Here's how the part is built. I have some questions about the finished solid (model axes, mm). Face numbers are marked on the shaded views. A direction names the side the tool comes from. Round coordinates to 2 decimals unless told otherwise and drop trailing zeros. Loops run counter-clockwise (first coordinate to the right, second up) from the corner with the lowest first, then second, coordinate; pieces in that order, holes last. Notation, with made-up numbers: (-0.75, 24.25) - (23.25, 24.25) arc R14 ccw to (23.25, 38.25) - close; hole circle Ø10 at (34, 70.5). An arc over 180 degrees is marked (long way). Answer as a JSON object with one key per item and string values. Group by question number.
1) Will these pins go through, and if not, where does the flat tip stop? P1, Ø1.8, axis at x = 6, z = 7, coming from the +Y side; P2, Ø6, axis at x = 10.5, y = 6, coming from the +Z side; P3, Ø1, axis at x = 2.5, z = 5.5, coming from the +Y side.
2) I want a section at C-C, the plane x = 5.95. Please give me the cut outline in (y, z).
3) If I drill on line 1 along Z through (x, y) = (7.5, 4.5); line 2 along Y through (x, z) = (7.25, 1.5); line 3 along Y through (x, z) = (5, 7), over which ranges is the centre line in solid material (lowest first)? Write a range as [from, to].
4) I want a section at B-B, the plane y = 3. Please give me the cut outline in (x, z), then the cut area to 3 significant figures.
5) I want a section at A-A, the plane x = 9.5. Please give me the cut outline in (y, z).
6) I want a section at D-D, the plane y = 5. Please give me the cut outline in (x, z), then the cut area to 3 significant figures.
7) Which directions (+Z, -Z, +X, -X, +Y, -Y) give clear straight access to the entire face, cutting with the end or side of a thin tool? Please do the marked faces 1 and 2.
from build123d import *

# Parameters (mm, degrees)
CROQUIS1_W              = 11.9
CROQUIS1_H              = 9.3
SALIENTE_EXTRUIR1_DEPTH = 10
SALIENTE_EXTRUIR2_DEPTH = 10
SALIENTE_EXTRUIR3_DEPTH = 16.3
CROQUIS6_W              = 10.1
CROQUIS6_H              = 0.1
CORTAR_EXTRUIR1_DEPTH   = 0.1
CROQUIS7_W              = 0.1
CROQUIS7_H              = 8.2
CORTAR_EXTRUIR2_DEPTH   = 0.1
CROQUIS8_W              = 0.1
CROQUIS8_H              = 8.2
CORTAR_EXTRUIR3_DEPTH   = 0.1
CROQUIS9_W              = 10.1
CROQUIS9_H              = 0.1
CORTAR_EXTRUIR4_DEPTH   = 0.1


with BuildPart() as part:
    # Croquis1 → Saliente-Extruir1 (new body)
    with BuildSketch(Plane(origin=(0, 0, 0), x_dir=(1, 0, 0), z_dir=(0, 1, 0))):
        with Locations((5.95, 4.65)):
            Rectangle(CROQUIS1_W, CROQUIS1_H)
    extrude(amount=SALIENTE_EXTRUIR1_DEPTH)

    # Croquis2 → Saliente-Extruir2 (add)
    with BuildSketch(Plane.XY):
        with BuildLine():
            Line((4.831966011, 6), (7.068033989, 6))
            ThreePointArc((7.068033989, 6), (5.95, 3.5), (4.831966011, 6))
        make_face()
    extrude(amount=SALIENTE_EXTRUIR2_DEPTH)

    # Croquis3 → Saliente-Extruir3 (add)
    with BuildSketch(Plane(origin=(0, 0, -9.3), x_dir=(-1, 0, 0), z_dir=(0, 0, -1))):
        with BuildLine():
            Line((-11, 10), (-0.9, 10))
            ThreePointArc((-0.9, 10), (-0.263603897, 9.736396103), (0, 9.1))
            Line((0, 9.1), (0, 0.9))
            ThreePointArc((0, 0.9), (-0.263603897, 0.263603897), (-0.9, 0))
            Line((-0.9, 0), (-11, 0))
            ThreePointArc((-11, 0), (-11.636396103, 0.263603897), (-11.9, 0.9))
            Line((-11.9, 0.9), (-11.9, 9.1))
            ThreePointArc((-11.9, 9.1), (-11.636396103, 9.736396103), (-11, 10))
        make_face()
    extrude(amount=SALIENTE_EXTRUIR3_DEPTH)

    # Croquis6 → Cortar-Extruir1 (cut)
    with BuildSketch(Plane(origin=(0, 10, 0), x_dir=(1, 0, 0), z_dir=(0, 1, 0))):
        with Locations((5.95, 9.35)):
            Rectangle(CROQUIS6_W, CROQUIS6_H)
    extrude(amount=-CORTAR_EXTRUIR1_DEPTH, mode=Mode.SUBTRACT)

    # Croquis7 → Cortar-Extruir2 (cut)
    with BuildSketch(Plane(origin=(11.9, 0, 0), x_dir=(0, 0, -1), z_dir=(1, 0, 0))):
        with Locations((9.35, 5)):
            Rectangle(CROQUIS7_W, CROQUIS7_H)
    extrude(amount=-CORTAR_EXTRUIR2_DEPTH, mode=Mode.SUBTRACT)

    # Croquis8 → Cortar-Extruir3 (cut)
    with BuildSketch(Plane.ZY):
        with Locations((-9.35, 5)):
            Rectangle(CROQUIS8_W, CROQUIS8_H)
    extrude(amount=-CORTAR_EXTRUIR3_DEPTH, mode=Mode.SUBTRACT)

    # Croquis9 → Cortar-Extruir4 (cut)
    with BuildSketch(Plane.XZ):
        with Locations((5.95, -9.35)):
            Rectangle(CROQUIS9_W, CROQUIS9_H)
    extrude(amount=-CORTAR_EXTRUIR4_DEPTH, mode=Mode.SUBTRACT)


solid = part.part
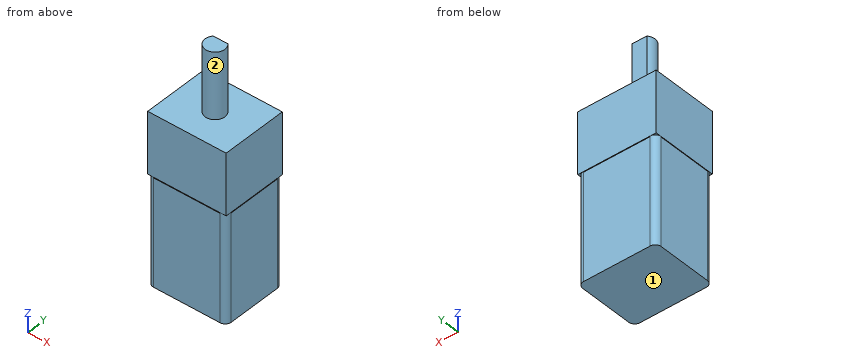
Outcome:
{
 "1": {"P1": "y = 6", "P2": "z = 0", "P3": "through"},
 "2": {"outline": "(0, -25.6) - (10, -25.6) - (10, -9.4) - (9.9, -9.4) - (9.9, -9.3) - (10, -9.3) - (10, 0) - (6, 0) - (6, 10) - (3.5, 10) - (3.5, 0) - (0, 0) - (0, -9.3) - (0.1, -9.3) - (0.1, -9.4) - (0, -9.4) - close"},
 "3": {"line 1": "[-25.6, 0]", "line 2": "[4.25, 5.75]", "line 3": "[3.84, 6]"},
 "4": {"outline": "(0, -25.6) - (11.9, -25.6) - (11.9, -9.4) - (11.8, -9.4) - (11.8, -9.3) - (11.9, -9.3) - (11.9, 0) - (0, 0) - (0, -9.3) - (0.1, -9.3) - (0.1, -9.4) - (0, -9.4) - close", "area": "305 mm^2"},
 "5": {"outline": "(0, -25.6) - (10, -25.6) - (10, -9.4) - (9.9, -9.4) - (9.9, -9.3) - (10, -9.3) - (10, 0) - (0, 0) - (0, -9.3) - (0.1, -9.3) - (0.1, -9.4) - (0, -9.4) - close"},
 "6": {"outline": "(0, -25.6) - (11.9, -25.6) - (11.9, -9.4) - (11.8, -9.4) - (11.8, -9.3) - (11.9, -9.3) - (11.9, 0) - (7.45, 0) - (7.45, 10) - (4.45, 10) - (4.45, 0) - (0, 0) - (0, -9.3) - (0.1, -9.3) - (0.1, -9.4) - (0, -9.4) - close", "area": "335 mm^2"},
 "7": {"face 1": "-Z, +X, -X, +Y, -Y", "face 2": "+Z"}
}
